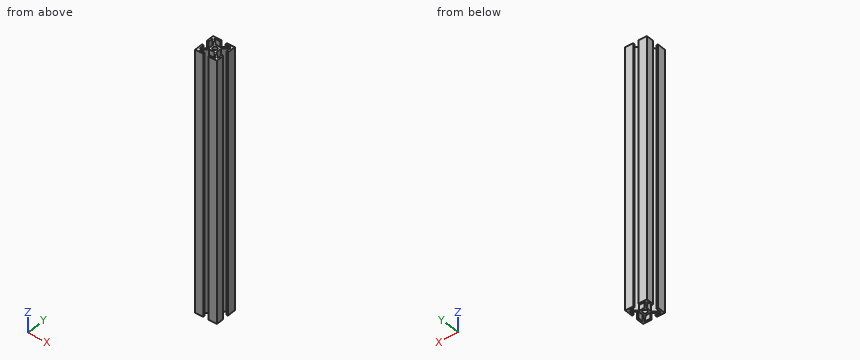
Autodesk Inventor part; units mm, degrees
ref_plane "YZ Plane" through (0, 0, 0) normal (1, 0, 0) x (0, 1, 0)
ref_plane "XZ Plane" through (0, 0, 0) normal (0, 1, 0) x (-1, 0, 0)
ref_plane "XY Plane" through (0, 0, 0) normal (0, 0, 1) x (1, 0, 0)
sketch "Sketch1" plane through (0, 0, 0) normal (0, 0, 1) x (1, 0, 0)
  line L0 (-12.7, 12.7) -> (12.7, 12.7)
  line L1 (12.7, 12.7) -> (12.7, -12.7)
  line L2 (12.7, -12.7) -> (-12.7, -12.7)
  line L3 (-12.7, -12.7) -> (-12.7, 12.7)
  point P0 (0, 0)
  dimension "d0" = 25.4
  dimension "d1" = 25.4
  dimension "d2" = 12.7
  dimension "d3" = 12.7
extrude "Extrusion1" add sketch "Sketch1" along normal blind 304.8
sketch "Sketch2" plane through (0, 0, 304.8) normal (0, 0, 1) x (1, 0, 0)
  circle A0 centre (0, 0) radius 2.54
  line L0 (-4.5085, 4.5085) -> (4.5085, 4.5085)
  line L1 (-4.5085, -4.5085) -> (4.5085, -4.5085)
  line L2 (4.5085, 4.5085) -> (4.5085, -4.5085)
  line L3 (-4.5085, 4.5085) -> (-4.5085, -4.5085)
  line L4 (-3.0896, 4.5085) -> (-11.2811, 12.7)
  line L5 (-4.5085, 3.0537) -> (-12.7, 11.2452)
  line L6 (12.7, 12.7) -> (-12.7, 12.7)
  line L7 (-12.7, 12.7) -> (-12.7, 4.0005)
  line L8 (-10.668, 4.0005) -> (-10.668, 9.2132)
  line L9 (-9.2491, 10.668) -> (-3.3655, 10.668)
  line L10 (-12.7, 12.7) -> (-3.3655, 12.7)
  line L11 (-2.7305, 11.303) -> (-2.7305, 12.065)
  line L12 (-12.065, 3.3655) -> (-11.303, 3.3655)
  arc A1 (-12.7, 4.0005) -> (-12.065, 3.3655) centre (-12.065, 4.0005) ccw
  arc A2 (-11.303, 3.3655) -> (-10.668, 4.0005) centre (-11.303, 4.0005) ccw
  arc A3 (-3.3655, 10.668) -> (-2.7305, 11.303) centre (-3.3655, 11.303) ccw
  arc A4 (-2.7305, 12.065) -> (-3.3655, 12.7) centre (-3.3655, 12.065) ccw
  arc A5 (-3.3655, -11.303) -> (-4.0005, -10.668) centre (-4.0005, -11.303) ccw
  line L13 (-3.3655, -12.065) -> (-3.3655, -11.303)
  arc A6 (-4.0005, -12.7) -> (-3.3655, -12.065) centre (-4.0005, -12.065) ccw
  line L14 (-3.0537, -4.5085) -> (-11.2452, -12.7)
  line L15 (-10.668, -9.2491) -> (-10.668, -3.3655)
  line L16 (-4.5085, -3.0896) -> (-12.7, -11.2811)
  line L17 (-12.7, -12.7) -> (-12.7, -3.3655)
  arc A7 (-10.668, -3.3655) -> (-11.303, -2.7305) centre (-11.303, -3.3655) ccw
  line L18 (-11.303, -2.7305) -> (-12.065, -2.7305)
  arc A8 (-12.065, -2.7305) -> (-12.7, -3.3655) centre (-12.065, -3.3655) ccw
  line L19 (-4.0005, -10.668) -> (-9.2132, -10.668)
  line L20 (-12.7, -12.7) -> (-4.0005, -12.7)
  arc A9 (11.303, -3.3655) -> (10.668, -4.0005) centre (11.303, -4.0005) ccw
  line L21 (12.065, -3.3655) -> (11.303, -3.3655)
  arc A10 (12.7, -4.0005) -> (12.065, -3.3655) centre (12.065, -4.0005) ccw
  line L22 (4.5085, -3.0537) -> (12.7, -11.2452)
  line L23 (9.2491, -10.668) -> (3.3655, -10.668)
  line L24 (3.0896, -4.5085) -> (11.2811, -12.7)
  line L25 (12.7, -12.7) -> (3.3655, -12.7)
  arc A11 (3.3655, -10.668) -> (2.7305, -11.303) centre (3.3655, -11.303) ccw
  line L26 (2.7305, -11.303) -> (2.7305, -12.065)
  arc A12 (2.7305, -12.065) -> (3.3655, -12.7) centre (3.3655, -12.065) ccw
  line L27 (10.668, -4.0005) -> (10.668, -9.2132)
  line L28 (12.7, -12.7) -> (12.7, -4.0005)
  arc A13 (3.3655, 11.303) -> (4.0005, 10.668) centre (4.0005, 11.303) ccw
  line L29 (3.3655, 12.065) -> (3.3655, 11.303)
  arc A14 (4.0005, 12.7) -> (3.3655, 12.065) centre (4.0005, 12.065) ccw
  line L30 (3.0537, 4.5085) -> (11.2452, 12.7)
  line L31 (10.668, 9.2491) -> (10.668, 3.3655)
  line L32 (4.5085, 3.0896) -> (12.7, 11.2811)
  line L33 (12.7, 12.7) -> (12.7, 3.3655)
  arc A15 (10.668, 3.3655) -> (11.303, 2.7305) centre (11.303, 3.3655) ccw
  line L34 (11.303, 2.7305) -> (12.065, 2.7305)
  arc A16 (12.065, 2.7305) -> (12.7, 3.3655) centre (12.065, 3.3655) ccw
  line L35 (4.0005, 10.668) -> (9.2132, 10.668)
  line L36 (12.7, 12.7) -> (4.0005, 12.7)
  line L37 (-4.5085, 3.0537) -> (-4.5085, 4.5085)
  line L38 (-3.0896, 4.5085) -> (-4.5085, 4.5085)
  line L39 (-12.7, -12.7) -> (-4.0005, -12.7)
  line L40 (-4.0005, -10.668) -> (-9.2132, -10.668)
  line L41 (-10.668, -9.2491) -> (-10.668, -3.3655)
  line L42 (-12.7, -12.7) -> (-12.7, -3.3655)
  line L43 (-11.303, -2.7305) -> (-12.065, -2.7305)
  arc A17 (-10.668, -3.3655) -> (-11.303, -2.7305) centre (-11.303, -3.3655) ccw
  arc A18 (-12.065, -2.7305) -> (-12.7, -3.3655) centre (-12.065, -3.3655) ccw
  line L44 (-4.5085, -3.0896) -> (-4.5085, -4.5085)
  line L45 (-4.5085, -3.0896) -> (-12.7, -11.2811)
  line L46 (-3.0537, -4.5085) -> (-4.5085, -4.5085)
  line L47 (-3.0537, -4.5085) -> (-11.2452, -12.7)
  line L48 (-4.5085, -4.5085) -> (-4.5085, 4.5085)
  circle A19 centre (0, 0) radius 2.54
  line L49 (-4.5085, -4.5085) -> (4.5085, -4.5085)
  line L50 (-3.3655, -12.065) -> (-3.3655, -11.303)
  arc A20 (-4.0005, -12.7) -> (-3.3655, -12.065) centre (-4.0005, -12.065) ccw
  arc A21 (-3.3655, -11.303) -> (-4.0005, -10.668) centre (-4.0005, -11.303) ccw
  line L51 (12.7, -12.7) -> (12.7, -4.0005)
  line L52 (10.668, -4.0005) -> (10.668, -9.2132)
  line L53 (9.2491, -10.668) -> (3.3655, -10.668)
  line L54 (12.7, -12.7) -> (3.3655, -12.7)
  line L55 (2.7305, -11.303) -> (2.7305, -12.065)
  arc A22 (3.3655, -10.668) -> (2.7305, -11.303) centre (3.3655, -11.303) ccw
  arc A23 (2.7305, -12.065) -> (3.3655, -12.7) centre (3.3655, -12.065) ccw
  line L56 (3.0896, -4.5085) -> (4.5085, -4.5085)
  line L57 (3.0896, -4.5085) -> (11.2811, -12.7)
  line L58 (4.5085, -3.0537) -> (4.5085, -4.5085)
  line L59 (4.5085, -3.0537) -> (12.7, -11.2452)
  line L60 (4.5085, -4.5085) -> (-4.5085, -4.5085)
  circle A24 centre (0, 0) radius 2.54
  line L61 (4.5085, -4.5085) -> (4.5085, 4.5085)
  line L62 (12.065, -3.3655) -> (11.303, -3.3655)
  arc A25 (12.7, -4.0005) -> (12.065, -3.3655) centre (12.065, -4.0005) ccw
  arc A26 (11.303, -3.3655) -> (10.668, -4.0005) centre (11.303, -4.0005) ccw
  line L63 (12.7, 12.7) -> (4.0005, 12.7)
  line L64 (4.0005, 10.668) -> (9.2132, 10.668)
  line L65 (10.668, 9.2491) -> (10.668, 3.3655)
  line L66 (12.7, 12.7) -> (12.7, 3.3655)
  line L67 (11.303, 2.7305) -> (12.065, 2.7305)
  arc A27 (10.668, 3.3655) -> (11.303, 2.7305) centre (11.303, 3.3655) ccw
  arc A28 (12.065, 2.7305) -> (12.7, 3.3655) centre (12.065, 3.3655) ccw
  line L68 (4.5085, 3.0896) -> (4.5085, 4.5085)
  line L69 (4.5085, 3.0896) -> (12.7, 11.2811)
  line L70 (3.0537, 4.5085) -> (4.5085, 4.5085)
  line L71 (3.0537, 4.5085) -> (11.2452, 12.7)
  line L72 (4.5085, 4.5085) -> (4.5085, -4.5085)
  circle A29 centre (0, 0) radius 2.54
  line L73 (4.5085, 4.5085) -> (-4.5085, 4.5085)
  line L74 (3.3655, 12.065) -> (3.3655, 11.303)
  arc A30 (4.0005, 12.7) -> (3.3655, 12.065) centre (4.0005, 12.065) ccw
  arc A31 (3.3655, 11.303) -> (4.0005, 10.668) centre (4.0005, 11.303) ccw
  point P0 (-12.7, 3.3655)
  point P1 (-2.7305, 12.7)
  point P2 (-3.3655, -12.7)
  point P3 (-12.7, -2.7305)
  point P4 (12.7, -3.3655)
  point P5 (2.7305, -12.7)
  point P6 (3.3655, 12.7)
  point P7 (12.7, 2.7305)
  point P8 (-3.3655, -12.7)
  point P9 (-12.7, -2.7305)
  point P10 (12.7, -3.3655)
  point P11 (2.7305, -12.7)
  point P12 (3.3655, 12.7)
  point P13 (12.7, 2.7305)
  dimension "d6" = 5.08
  dimension "d7" = 9.017
  dimension "d8" = 4.5085
  dimension "d9" = 4.5085
  dimension "d10" = 4.5085
  dimension "d11" = 2.032
  dimension "d12" = 1.0033
  dimension "d13" = 135
  dimension "d17" = 9.3345
  dimension "d19" = 2.032
  dimension "d20" = 2.032
  dimension "d21" = 0.635
  dimension "d22" = 9.3345
  dimension "d25" = 360
  dimension "d29" = 360
extrude "Extrusion2" cut sketch "Sketch2" against normal blind 1219.2 contours L3 L5 L7 L6 L4 L0 | L0 L2 L1 L3 | L30 L6 L33 L32 L2 L0 | L4 L6 A4 L11 A3 L9 | L3 L1 L14 L20 L17 L16 | L8 A2 L12 A1 L7 L5 | L35 A13 L29 A14 L6 L30 | L16 L17 A8 L18 A7 L15 | L22 L28 L25 L24 L1 L2 | L32 L33 A16 L34 A15 L31 | L19 A5 L13 A6 L20 L14 | L27 A9 L21 A10 L28 L22 | L24 L25 A12 L26 A11 L23 keep common part
equation "\"d22\" = d17"
properties part number "Handle Holding PIECE"
Check sheet for the modelled part. Datum: model origin and axes. Units: mm. Give positions to 0.01 mm unless a question says otherwise; leave off trailing zeros. Loops run counter-clockwise (first coordinate to the right, second up) from the corner with the lowest first, then second, coordinate; pieces in that order, holes last. Notation, with made-up numbers: M -5.5,86 L 14.5,86 A15 cw 14.5,106 Z; hole C 23.5,21.25 d2. An arc over 180 degrees is marked long. Answer as a JSON object with one key per item and string values. Group by question number.
Q1. Go/stop test with flat-tipped pins: P1, Ø8, axis at x = 5.5, y = -2.5, coming from the -Z side; P2, Ø1.8, axis at y = 1, z = 100, coming from the +X side; P3, Ø1.8, axis at x = -1, z = 199.5, coming from the +Y side. Record where each tip stops, or that it passes through.
Q2. Material ranges on line 1 along Y through (x, z) = (0, 181); line 2 along Y through (x, z) = (-5.5, 185); line 3 along Y through (x, z) = (6.25, 169), recorded low to high. Write a range as [from, to].
Q3. Cross-section at A-A on y = 0. Record the cut outline in (x, z).
Evaluation:
{
 "1": {"P1": "stops at z = 0", "P2": "stops at x = 4.51", "P3": "stops at y = 4.51"},
 "2": {"line 1": "y = [-4.51, -2.54], [2.54, 4.51]", "line 2": "y = [-12.7, -10.67], [-6.95, -4.08], [4.05, 6.92], [10.67, 12.7]", "line 3": "y = [-12.7, -10.67], [-7.67, -4.8], [4.83, 7.7], [10.67, 12.7]"},
 "3": {"outline": "M -4.51,0 L -2.54,0 L -2.54,304.8 L -4.51,304.8 Z; M 2.54,0 L 4.51,0 L 4.51,304.8 L 2.54,304.8 Z"}
}
